Design review of the part shown in the three views and the two pictorial views. Dimensions are in mm from the part's minimum x, y and z. A direction names the side the tool comes from. Give positions to 0.01 mm unless a question says otherwise; leave off trailing zeros. Write each loop counter-clockwise with the first axis right and the second up, starting at its lowest first coordinate (ties: lowest second). Pieces come first, ordered by that corner, then holes.
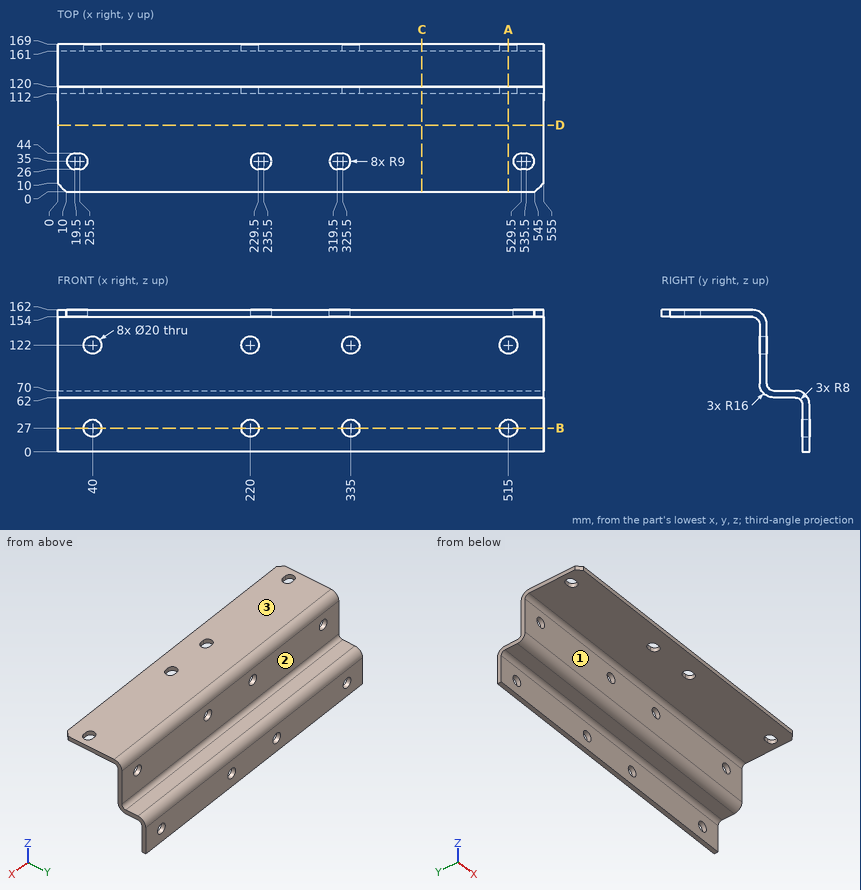
(1) Tool access review of the marked faces 1, 2 and 3: name each direction out of +Z, -Z, +X, -X, +Y, -Y from which nothing blocks a thin tool from reaching the whole face with its end or side.
Resolved:
face 1: -Z, +X, -X, -Y
face 2: +Z, +X, -X, +Y
face 3: +Z, +X, -X, +Y, -Y
(2) Consider section A-A, the plane x = 515. Give the boundary of the cut face in (y, z).
Resolved:
outline: (0, 154) - (104, 154) arc R8 cw to (112, 146) - (112, 132) - (120, 132) - (120, 146) arc R16 ccw to (104, 162) - (0, 162) - close; (112, 78) arc R16 ccw to (128, 62) - (153, 62) arc R8 cw to (161, 54) - (161, 37) - (169, 37) - (169, 54) arc R16 ccw to (153, 70) - (128, 70) arc R8 cw to (120, 78) - (120, 112) - (112, 112) - close; (161, 0) - (169, 0) - (169, 17) - (161, 17) - close
(3) Clearance check with flat-ended pins moving along their axes: P1, Ø1.5, axis at x = 481, z = 80, coming from the +Y side; P2, Ø12.5, axis at x = 401.5, y = 137, coming from the +Z side; P3, Ø12.5, axis at x = 345.5, y = 143.5, coming from the -Z side; P4, Ø16, axis at x = 515, z = 27, coming from the -Y side. State where each tip first meets the part, or that it passes through.
Resolved:
P1: stops at y = 120
P2: stops at z = 70
P3: stops at z = 62
P4: passes through
(4) Consider section C-C, the plane x = 416. Give the boundary of the cut face in (y, z), then the cut area to 3 significant figures.
Resolved:
outline: (0, 154) - (104, 154) arc R8 cw to (112, 146) - (112, 78) arc R16 ccw to (128, 62) - (153, 62) arc R8 cw to (161, 54) - (161, 0) - (169, 0) - (169, 54) arc R16 ccw to (153, 70) - (128, 70) arc R8 cw to (120, 78) - (120, 146) arc R16 ccw to (104, 162) - (0, 162) - close
area: 2,460 mm2
(5) Consider section D-D, the plane y = 76.5. Give the boundary of the cut face in (x, z), then the cut area to 3 significant figures.
Resolved:
outline: (0, 154) - (555, 154) - (555, 162) - (0, 162) - close
area: 4,440 mm2
(6) Consider section B-B, the plane z = 27. Give the boundary of the cut face in (x, y), then the cut area to 3 significant figures.
Resolved:
outline: (0, 161) - (30, 161) - (30, 169) - (0, 169) - close; (50, 161) - (210, 161) - (210, 169) - (50, 169) - close; (230, 161) - (325, 161) - (325, 169) - (230, 169) - close; (345, 161) - (505, 161) - (505, 169) - (345, 169) - close; (525, 161) - (555, 161) - (555, 169) - (525, 169) - close
area: 3,800 mm2
(7) To check wall thickness, follow L1, parallel to X at y = 163, z = 27; L2, parallel to Y at x = 168.5, z = 49.5; L3, parallel to Y at x = 441, z = 102.5. State the ranges of each line that lie inside material, in increasing order.
Resolved:
L1: x = 0 to 30, 50 to 210, 230 to 325, 345 to 505, 525 to 555
L2: y = 161 to 169
L3: y = 112 to 120
